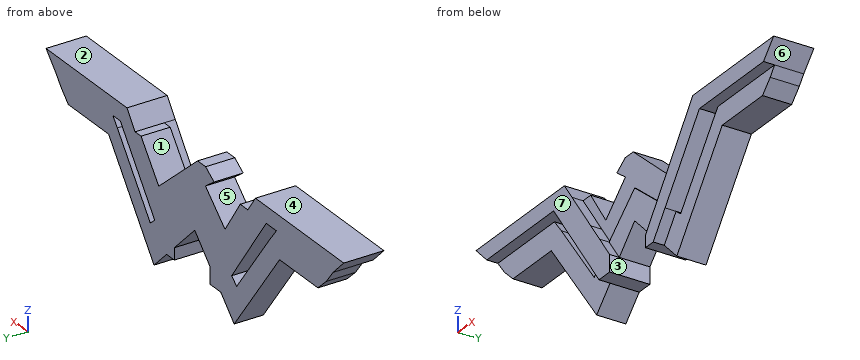
```python
from build123d import *

# Parameters (mm, degrees)
F1_DEPTH = 5.08
F2_DEPTH = 7.0104
F3_DEPTH = 5.334


with BuildPart() as f1:
    # F0 (on Front) → F1 (new body)
    with BuildSketch(Plane.XZ):
        Polygon((-40.062314, 7.287229), (-37.179609, 4.422599), (-21.960379, 4.422599), (-19.214497, 4.422599), (-9.926813, -8.524094), (-7.009587, -12.590599), (-4.146443, -12.590599), (-4.146443, -9.682406), (-6.864069, -5.894135), (-9.225641, -2.60219), (-14.265077, 4.422599), (-16.320102, 7.287229), align=None)
        Polygon((8.418841, -6.8194), (5.47293, -10.858879), (5.47293, -12.923377), (7.56991, -12.923377), (10.741626, -8.700894), (19.999054, 3.623457), (21.996683, 3.623457), (37.222218, 3.623457), (39.969709, 6.618017), (18.218485, 6.618017), (16.034611, 3.623457), (10.868541, -3.460336), align=None)
        Polygon((-35.363599, 2.096692), (-33.117508, 0), (-22.81333, 0), (-10.609382, -16.247032), (-7.009587, -12.590599), (-9.926813, -8.524094), (-11.275736, -9.682406), (-20.123599, 2.096692), align=None)
        Polygon((-37.179609, 4.422599), (-35.363599, 2.096692), (-20.123599, 2.096692), (-21.960379, 4.422599), align=None)
        Polygon((-12.233077, 4.422599), (-14.265077, 4.422599), (-9.225641, -2.60219), (-8.147482, -1.614384), align=None)
        Polygon((-9.225641, -2.60219), (-6.864069, -5.894135), (0, 0), (8.418841, -6.8194), (10.868541, -3.460336), (9.668322, -2.531922), (-0.779053, 6.436089), (-2.935238, 6.436089), (-5.197461, 4.922159), (-2.880355, 3.211346), (-8.147482, -1.614384), align=None)
        Polygon((-6.864069, -5.894135), (-4.146443, -9.682406), (0, -5.470725), (5.47293, -10.858879), (8.418841, -6.8194), (0, 0), align=None)
        Polygon((10.741626, -8.700894), (7.56991, -12.923377), (10.945859, -16.247032), (23.149807, 0), (33.976993, 0), (36.041207, 2.096692), (20.801207, 2.096692), (11.953345, -9.682406), align=None)
        Polygon((21.996683, 3.623457), (20.801207, 2.096692), (36.041207, 2.096692), (37.222218, 3.623457), align=None)
        Polygon((9.668322, -2.531922), (10.868541, -3.460336), (16.034611, 3.623457), (14.429741, 3.623457), align=None)
    extrude(amount=F1_DEPTH)

    # F0 (on Front) → F2 (join)
    with BuildSketch(Plane.XZ):
        Polygon((8.418841, -6.8194), (5.47293, -10.858879), (5.47293, -12.923377), (7.56991, -12.923377), (10.741626, -8.700894), (19.999054, 3.623457), (21.996683, 3.623457), (37.222218, 3.623457), (39.969709, 6.618017), (18.218485, 6.618017), (16.034611, 3.623457), (10.868541, -3.460336), align=None)
        Polygon((-40.062314, 7.287229), (-37.179609, 4.422599), (-21.960379, 4.422599), (-19.214497, 4.422599), (-9.926813, -8.524094), (-7.009587, -12.590599), (-4.146443, -12.590599), (-4.146443, -9.682406), (-6.864069, -5.894135), (-9.225641, -2.60219), (-14.265077, 4.422599), (-16.320102, 7.287229), align=None)
    extrude(amount=F2_DEPTH)

    # F0 (on Front) → F3 (join)
    with BuildSketch(Plane.XZ):
        Polygon((-6.864069, -5.894135), (-4.146443, -9.682406), (0, -5.470725), (5.47293, -10.858879), (8.418841, -6.8194), (0, 0), align=None)
    extrude(amount=F3_DEPTH)


solid = f1.part
```
Part model, mm, in its own coordinate system. Face numbers are marked on the shaded views. A direction names the side the tool comes from. Round coordinates to 2 decimals unless told otherwise and drop trailing zeros. Loops run counter-clockwise (first coordinate to the right, second up) from the corner with the lowest first, then second, coordinate; pieces in that order, holes last.
1. Slice it at C-C (y = -4.25). Count the separate pieces of the cut face and the enclosed holes in it, and give its area (3 significant figures).
Solutions:
separate pieces: 1
enclosed holes: 2
area: 741 mm2
2. Two-plate mould, pull along Z, no slides. Class the marked faces 4, 5, 6 and 7: pulls with the +Z half, pulls with the -Z half, needs draft (parallel to the pull), parting line crosses it, or undercut.
Solutions:
face 4: pulls with the +Z half
face 5: undercut
face 6: pulls with the -Z half
face 7: needs draft
3. Drill centre lines: line 1 along X through (y, z) = (-1.25, -3.5); line 2 along X through (y, z) = (-1, -4); line 3 along X through (y, z) = (-3.5, -9). Where is each one in solid material? Low to high.
Solutions:
line 1: x = -20.18 to -15.92, -13.53 to 14.65, 16.6 to 20.52
line 2: x = -19.81 to -15.54, -13.17 to 14.27, 16.22 to 20.15
line 3: x = -16.05 to -11.79, -10.48 to -3.47, 3.58 to 11.11, 12.47 to 16.39
4. Slice it at A-A (z = -7.5). Give the cut face in (x, y), and give its area (3 significant figures).
Solutions:
outline: (-17.18, -5.08) - (-12.92, -5.08) - (-12.92, 0) - (-17.18, 0) - close; (-10.66, -7.01) - (-5.71, -7.01) - (-5.71, -5.33) - (-2, -5.33) - (-2, 0) - (-10.66, 0) - close; (2.06, -5.33) - (7.92, -5.33) - (7.92, -7.01) - (11.64, -7.01) - (11.64, 0) - (2.06, 0) - close; (13.59, -5.08) - (17.52, -5.08) - (17.52, 0) - (13.59, 0) - close
area: 153 mm2
5. Slice it at D-D (x = -34). Give the cut face in (y, z).
Solutions:
outline: (-7.01, 4.42) - (-5.08, 4.42) - (-5.08, 0.82) - (0, 0.82) - (0, 7.29) - (-7.01, 7.29) - close
6. 3-axis set-ups, long thin cutter, end or side, ignore diameter. For the marked faces 1, 2 and 3: which of +Z, -Z, +X, -X, +Y, -Y reach the whole face in a straight line?
Solutions:
face 1: +Z, +Y, -Y
face 2: +Z, +X, +Y, -Y
face 3: -Z, +Y, -Y
7. Flat gauge pins, fed straight in: pin 1 (3 mm diameter, centred on x = -3.5, y = -3, fed in from -Z); pin 2 (1 mm diameter, centred on y = -4, z = -12.5, fed in from -X); pin 3 (8 mm diameter, centred on x = -25.5, z = -3, fed in from -Y); pin 4 (1 mm diameter, centred on x = 15.5, z = 4.5, fed in from -Y). Where does each tip first touch, or does it go through?
Solutions:
pin 1: stops at z = -12.59
pin 2: stops at x = -13.8
pin 3: stops at y = -5.08
pin 4: passes through
8. Slice it at B-B (x = 30). Give the cut face in (y, z).
Solutions:
outline: (-7.01, 3.62) - (-5.08, 3.62) - (-5.08, 0) - (0, 0) - (0, 6.62) - (-7.01, 6.62) - close
